Check sheet for the drawn part. Datum: minimum x, y, z corner. Units: mm. Round coordinates to 2 decimals unless told otherwise and drop trailing zeros. Loops run counter-clockwise (first coordinate to the right, second up) from the corner with the lowest first, then second, coordinate; pieces in that order, holes last.
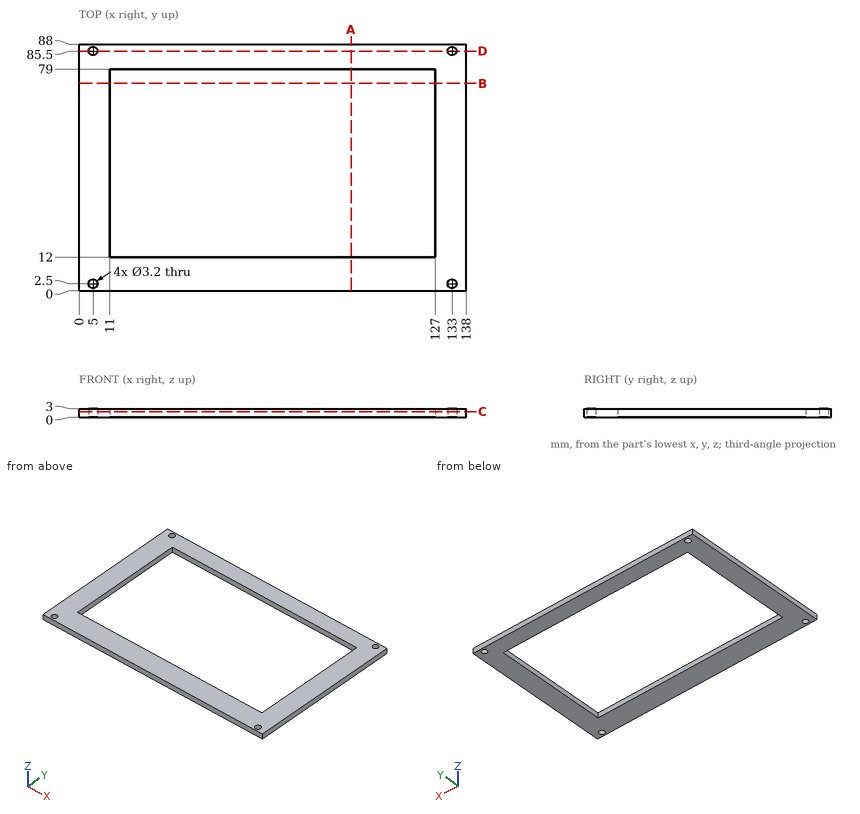
1) Sectioned sample at A-A, the plane x = 97. Record the cut outline in (y, z).
Report:
outline: (0, 0) - (12, 0) - (12, 3) - (0, 3) - close; (79, 0) - (88, 0) - (88, 3) - (79, 3) - close
2) Sectioned sample at D-D, the plane y = 85.5. Record the cut outline in (x, z), then the cut area to 3 significant figures.
Report:
outline: (0, 0) - (3.4, 0) - (3.4, 3) - (0, 3) - close; (6.6, 0) - (131.4, 0) - (131.4, 3) - (6.6, 3) - close; (134.6, 0) - (138, 0) - (138, 3) - (134.6, 3) - close
area: 395 mm2
3) Sectioned sample at B-B, the plane y = 74. Record the cut outline in (x, z), then the cut area to 3 significant figures.
Report:
outline: (0, 0) - (11, 0) - (11, 3) - (0, 3) - close; (127, 0) - (138, 0) - (138, 3) - (127, 3) - close
area: 66.0 mm2
4) Sectioned sample at C-C, the plane z = 2.05. Record the cut outline in (x, y), then the cut area to 3 significant figures.
Report:
outline: (0, 0) - (138, 0) - (138, 88) - (0, 88) - close; hole circle Ø3.2 at (5, 2.5); hole circle Ø3.2 at (5, 85.5); hole (11, 12) - (127, 12) - (127, 79) - (11, 79) - close; hole circle Ø3.2 at (133, 2.5); hole circle Ø3.2 at (133, 85.5)
area: 4,340 mm2
5) Scan lines: line 1 along X through (y, z) = (85.5, 1.75); line 2 along Y through (x, z) = (133, 2.3); line 3 along Y through (x, z) = (19, 0.8). Record each from-to range of solid material in increasing order.
Report:
line 1: x = 0 to 3.4, 6.6 to 131.4, 134.6 to 138
line 2: y = 0 to 0.9, 4.1 to 83.9, 87.1 to 88
line 3: y = 0 to 12, 79 to 88
6) Gauge pin test, flat end, axial feed: pin 1 (1.9 mm diameter, centred on x = 5, y = 2.5, fed in from -Z). Record the tip position at first contact, or that the pin passes through.
Report:
pin 1: passes through
